For this review, take the finished solid that the model builds, in its own axes (mm). A direction names the side the tool comes from. Coordinates: 2 decimals unless noted, no trailing zeros. Loops run counter-clockwise (first coordinate to the right, second up) from the corner with the lowest first, then second, coordinate; pieces in that order, holes last. Notation, with made-up numbers: (61.25, 33.25) -> (106.25, 33.25) arc R28 cw to (106.25, 56.25) -> close; hole circle Ø7 at (-35.5, -13). An arc over 180 degrees is marked (long way). One line per item, written item: value.
from build123d import *

# Parameters (mm, degrees)
F0_R     = 22.9132131763
F1_DEPTH = 40
F2_DEPTH = 400


# Not quite as in the source:
# - a feature names something its author has since deleted; it is built from what else it names


with BuildPart() as f1:
    # F0 (on Top) → F1 (new body)
    with BuildSketch(Plane.XY):
        with BuildLine():
            ThreePointArc((-599.9922642108, -94.5975626578), (-55.9908868153, -192.3217779419), (39.4396888844, 352.0866405113))
            ThreePointArc((39.4396888844, 352.0866405113), (-342.3269144878, 217.5704996833), (-599.9922642108, -94.5975626578))
        make_face()
        with Locations((-505.0551273235, -100.2501100564)):
            Circle(F0_R, mode=Mode.SUBTRACT)
        with Locations((-74.5249837637, -137.0074301958)):
            Circle(F0_R, mode=Mode.SUBTRACT)
        with Locations((28.9413593709, 293.3445572853)):
            Circle(F0_R, mode=Mode.SUBTRACT)
        with Locations((28.9413593709, 293.3445572853)):
            Circle(F0_R)
        with Locations((-74.5249837637, -137.0074301958)):
            Circle(F0_R)
        with Locations((-505.0551273235, -100.2501100564)):
            Circle(F0_R)
    extrude(amount=F1_DEPTH)

    # F0 (on Top) → F2 (join)
    with BuildSketch(Plane.XY):
        with Locations((-505.0551273235, -100.2501100564)):
            Circle(F0_R)
        with Locations((-74.5249837637, -137.0074301958)):
            Circle(F0_R)
        with Locations((28.9413593709, 293.3445572853)):
            Circle(F0_R)
    extrude(amount=-F2_DEPTH)


solid = f1.part
1. To check wall thickness, follow probe 1 along Z at (x, y) = (-362.5, -73); probe 2 along X at (y, z) = (-161.5, 16.5); probe 3 along X at (y, z) = (221, 18.5). State the ranges of each line that lie inside material, in increasing order. Write a range as from..to.
Return value:
probe 1: z = 0..40
probe 2: x = -541.33..-17.34
probe 3: x = -337.38..99.27
2. Insertion check: pin 1 Ø1 at (x, y) = (-430.5, 113) entering from -Z. The pin has a flat end and moves straight along its axis. Give the tip position at first contact, or say it passes through.
Return value:
pin 1: stops at z = 0
3. For faces 1 (the cylindrical face through (-494.482, -120.578, -197.2)), 2 (the flat face through (-171, 49, 40)), list the 3-axis set-ups (+Z, -Z, +X, -X, +Y, -Y) from which the entire face can be reached by the end or side of a thin tool; tool diameter is ignored.
Return value:
face 1: -Z
face 2: +Z, +X, -X, +Y, -Y
4. The part is to be moulded in two halves that separate along X. For faces 3 (the cylindrical face through (39.514, 273.017, -197.2)), 4 (the cylindrical face through (-337.61, 220.84, 19.72)), 5 (the cylindrical face through (-92.71, -150.95, -197.2)), 6 (the flat face through (29, 294, -400)), say which applies: pulls with the +X half, pulls with the -X half, needs draft (parallel to the pull), parting line crosses it, or undercut.
Return value:
face 3: parting line crosses it
face 4: pulls with the -X half
face 5: undercut
face 6: needs draft
5. Take a section at A-A, the plane z = -338. Give the boundary of the cut face in (x, y).
Return value:
outline: circle Ø45.83 at (-505.06, -100.25); circle Ø45.83 at (-74.52, -137.01); circle Ø45.83 at (28.94, 293.34)
6. Take a section at B-B, the plane y = 13. Give the boundary of the cut face in (x, z), and give its area (3 significant figures).
Return value:
outline: (-541.18, 0) -> (93.51, 0) -> (93.51, 40) -> (-541.18, 40) -> close
area: 25,400 mm2
7. Take a section at C-C, the plane x = -430. Give the boundary of the cut face in (y, z).
Return value:
outline: (-232.33, 0) -> (145.99, 0) -> (145.99, 40) -> (-232.33, 40) -> close
